For this review, take the finished solid that the model builds, in its own axes (mm). Give positions to 0.01 mm unless a question says otherwise; leave off trailing zeros. Order: outer loops, then holes, each group sorted by start corner. A loop starts at its lowest first (then second) coordinate and runs counter-clockwise, first axis right, second up. Notation, with made-up numbers: M 78.5,53 L 106.5,53 A17 ccw 106.5,59 Z; hole C 46.5,9 d10. An arc over 180 degrees is marked long. Use CSV: the item, a comma, the result in double quotes. Start each with the question number.
(1) Consider section B-B (z = -0.6). Write out the cut boundary in (x, y), and give its area (3 significant figures).
(2) Consider section A-A (y = 0). Write out the cut boundary in (x, z), and give its area (3 significant figures).
(3) Wall thickness on L1, parallel to X at y = 1.5, z = 0.3; L2, parallel to X at y = -3, z = -0.45; L3, parallel to Y at x = -0.5, z = 0.2: over which ranges is each line inside the solid? List them lowest first. Write a range as from..to.
```python
from build123d import *

# Parameters (mm, degrees)
HEX_SKETCH_R               = 4
HEX_2_DEPTH                = 1
HEX_CHAM_ID_SIZE           = 0.25
HEX_ROUND_DEPTH            = 8.702813339
HEX_ROUND_DEPTH_BACK       = 8.702813339
HEX_ROUND_SKETCH_OUTSIDE_W = 16.63
HEX_ROUND_SKETCH_OUTSIDE_H = 15.082
HEX_ROUND_SKETCH_OUTSIDE_R = 5.3


with BuildPart() as part:
    # Hex_Sketch → Hex 2 (new, symmetric)
    with BuildSketch(Plane.XY):
        Polygon((2.886751346, 5), (-2.886751346, 5), (-5.773502692, 0), (-2.886751346, -5), (2.886751346, -5), (5.773502692, 0), align=None)
        Circle(HEX_SKETCH_R, mode=Mode.SUBTRACT)
    extrude(amount=HEX_2_DEPTH, both=True)

    # Hex Cham OD_Sketch → Hex Cham OD (revolve, cut)
    with BuildSketch(Plane(origin=(0, 0, 0), x_dir=(1, 0, 0), z_dir=(0, 1, 0))):
        Polygon((-5.773502692, 1), (-5.773502692, 0.553418013), (-5, 1), align=None)
        Polygon((-5, -1), (-5.773502692, -1), (-5.773502692, -0.553418013), align=None)
    revolve(axis=Axis((0, 0, -5.304715554), (0, 0, 1)), mode=Mode.SUBTRACT)

    # Hex Cham ID
    hex_cham_id_edges = [part.edges().sort_by_distance(p)[0] for p in [
        (-4, 0, -1),
        (-4, 0, 1),
    ]]
    chamfer(hex_cham_id_edges, length=HEX_CHAM_ID_SIZE)

    # Hex Round_Sketch outside → Hex Round (cut, two sides: drawn at the far end of the back side and taken through both)
    with BuildSketch(Plane.XY.offset(-HEX_ROUND_DEPTH_BACK)):
        Rectangle(HEX_ROUND_SKETCH_OUTSIDE_W, HEX_ROUND_SKETCH_OUTSIDE_H)
        Circle(HEX_ROUND_SKETCH_OUTSIDE_R, mode=Mode.SUBTRACT)
    extrude(amount=HEX_ROUND_DEPTH + HEX_ROUND_DEPTH_BACK, mode=Mode.SUBTRACT)


solid = part.part
```
Check result:
1,outline,"M -5.21,-0.98 L -3.45,-4.02 A5.3 ccw -1.76,-5 L 1.76,-5 A5.3 ccw 3.45,-4.02 L 5.21,-0.98 A5.3 ccw 5.21,0.98 L 3.45,4.02 A5.3 ccw 1.76,5 L -1.76,5 A5.3 ccw -3.45,4.02 L -5.21,0.98 A5.3 ccw Z; hole C 0,0 d8"
1,area,"33.7 mm^2"
2,outline,"M -5.3,-0.83 L -5,-1 L -4.25,-1 L -4,-0.75 L -4,0.75 L -4.25,1 L -5,1 L -5.3,0.83 Z; M 4,-0.75 L 4.25,-1 L 5,-1 L 5.3,-0.83 L 5.3,0.83 L 5,1 L 4.25,1 L 4,0.75 Z"
2,area,"4.97 mm^2"
3,L1,"x = -4.91..-3.71, 3.71..4.91"
3,L2,"x = -4.04..-2.65, 2.65..4.04"
3,L3,"y = -5..-3.97, 3.97..5"
